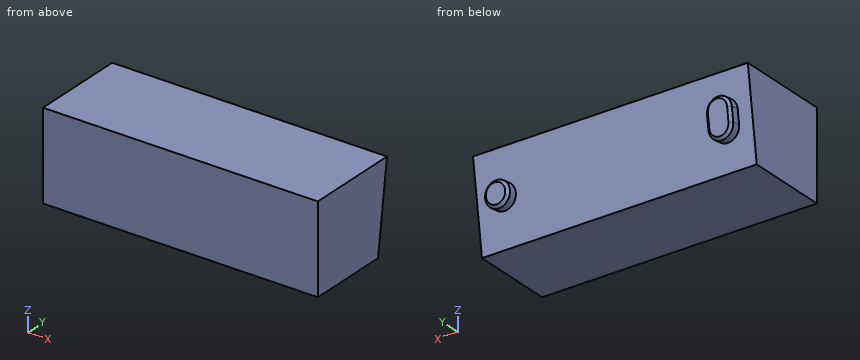
from build123d import *

# Parameters (mm, degrees)
EXTRUDE_1_DEPTH     = 16
CUT_EXTRUDE_1_DEPTH = 50
EXTRUDE_2_DEPTH     = 28.5
SKETCH_4_R          = 4.5
CUT_EXTRUDE_2_DEPTH = 28.5
EXTRUDE_3_DEPTH     = 50
EXTRUDE_START       = 4
SKETCH_6_R          = 4.5
EXTRUDE_4_DEPTH     = 4
CUT_EXTRUDE_3_DEPTH = 60
CHAMFER_1_SIZE      = 1


with BuildPart() as part:
    # 草图1 → 凸台-拉伸1 (new, symmetric)
    with BuildSketch(Plane.XY):
        with BuildLine():
            Line((-17, 0), (-17, -66.86388681))
            Line((-17, -66.86388681), (-20.5, -66.86388681))
            Line((-20.5, -66.86388681), (-20.5, 0))
            ThreePointArc((-20.5, 0), (0, 20.5), (20.5, 0))
            Line((20.5, 0), (20.5, -66.86388681))
            Line((20.5, -66.86388681), (17, -66.86388681))
            Line((17, -66.86388681), (17, 0))
            ThreePointArc((17, 0), (0, 17), (-17, 0))
        make_face()
    extrude(amount=EXTRUDE_1_DEPTH, both=True)

    # 草图2 → 切除-拉伸1 (cut, symmetric)
    with BuildSketch(Plane(origin=(0, 0, 0), x_dir=(0, 0, -1), z_dir=(1, 0, 0))):
        Polygon((16, -42.748653355), (-16, -38.251346645), (-16, -66.86388681), (16, -66.86388681), align=None)
    extrude(amount=CUT_EXTRUDE_1_DEPTH, both=True, mode=Mode.SUBTRACT)

    # 草图3 → 凸台-拉伸2 (add)
    with BuildSketch(Plane.ZY.offset(20.5)):
        Polygon((-16, -42.748653355), (16, -38.251346645), (16, -34.716950141), (-16, -39.214256851), align=None)
    extrude_2 = extrude(amount=EXTRUDE_2_DEPTH)

    # 镜向1: 凸台-拉伸2 across plane
    add(extrude_2.mirror(Plane(origin=(0, 0, 0), x_dir=(0, 0, 1), z_dir=(1, 0, 0))))

    # 草图4 → 切除-拉伸2 (cut)
    with BuildSketch(Plane(origin=(0, -36.249611102, 5.094550602), x_dir=(1, 0, 0), z_dir=(0, 0.9902680687415715, -0.13917310096005808))):
        with Locations(Location((40.5, 5.144617667, 0), (0, 0, 270))):
            Circle(SKETCH_4_R)
        with BuildLine():
            Line((-36, 7.644617667), (-36, 2.644617667))
            ThreePointArc((-36, 2.644617667), (-40.5, -1.855382333), (-45, 2.644617667))
            Line((-45, 2.644617667), (-45, 7.644617667))
            ThreePointArc((-45, 7.644617667), (-40.5, 12.144617667), (-36, 7.644617667))
        make_face()
    extrude(amount=-CUT_EXTRUDE_2_DEPTH, mode=Mode.SUBTRACT)

    # 草图8 → 切除-拉伸3 (cut, symmetric)
    with BuildSketch(Plane(origin=(0, 0, 0), x_dir=(0, 0, -1), z_dir=(1, 0, 0))):
        Polygon((16, -42.748653355), (-16, -38.251346645), (-16, 32.293524638), (16, 32.293524638), align=None)
    extrude(amount=CUT_EXTRUDE_3_DEPTH, both=True, mode=Mode.SUBTRACT)


with BuildPart() as body_2:
    # 草图5 → 凸台-拉伸3 (new, symmetric)
    with BuildSketch(Plane(origin=(0, 0, 0), x_dir=(0, 0, -1), z_dir=(1, 0, 0))):
        Polygon((16, -42.748653355), (-16, -38.251346645), (-16, -72.998653355), (16, -72.998653355), align=None)
    extrude(amount=EXTRUDE_3_DEPTH, both=True)

    # 草图6 → 凸台-拉伸4 (add)
    with BuildSketch(Plane(origin=(0, -39.715549343, 5.581656455), x_dir=(1, 0, 0), z_dir=(0, 0.9902680687415714, -0.139173100960058)).offset(EXTRUDE_START)):
        with Locations(Location((40.5, 5.144617667, 0), (0, 0, 90))):
            Circle(SKETCH_6_R)
        with BuildLine():
            Line((-36, 2.644617667), (-36, 7.644617667))
            ThreePointArc((-36, 7.644617667), (-40.5, 12.144617667), (-45, 7.644617667))
            Line((-45, 7.644617667), (-45, 2.644617667))
            ThreePointArc((-45, 2.644617667), (-40.5, -1.855382333), (-36, 2.644617667))
        make_face()
    extrude(amount=-EXTRUDE_4_DEPTH)

    # 倒角1
    chamfer_1_edges = [body_2.edges().sort_by_distance(p)[0] for p in [
        (-40.5, -35.496257755, 6.862289931),
        (-36, -36.470469462, -0.06958655),
        (-40.5, -37.444681169, -7.001463032),
        (-45, -36.470469462, -0.06958655),
        (40.5, -35.844190507, 4.386619759),
    ]]
    chamfer(chamfer_1_edges, length=CHAMFER_1_SIZE)


solid = body_2.part
Input: part model. Units: mm. Frame: model coordinates. Give positions to 0.01 mm unless a question says otherwise; leave off trailing zeros. Order: outer loops, then holes, each group sorted by start corner. A loop starts at its lowest first (then second) coordinate and runs counter-clockwise, first axis right, second up. Notation, with made-up numbers: (65, 63) -> (72, 63) arc R14 ccw to (72, 90) -> close; hole circle Ø1 at (80.5, -27.75). An arc over 180 degrees is marked (long way). Use one line per item in the form item = value.
1) Line query: probe 1 along Y at (x, z) = (-31.5, -4); probe 2 along Y at (x, z) = (18, -6.5). Output: solid intervals per line, ascending.
Response values:
probe_1 = -73 to -41.06
probe_2 = -73 to -41.41
2) First-contact query: pin 1 Ø12 at (x, z) = (22.5, -1.5) entering from +Y; pin 2 Ø10 at (x, z) = (-21.5, 0.5) entering from +Y; pin 3 Ø10 at (x, z) = (32.5, 6) entering from +Y. Flat tips, straight axial feed; report the tip coordinate or a pass-through.
Response values:
pin_1 = -39.87
pin_2 = -39.73
pin_3 = -38.95
3) Section A-A, the plane x = 11. Return loops of the section in (y, z), and give its area (3 significant figures).
Response values:
outline = (-73, -16) -> (-42.75, -16) -> (-38.25, 16) -> (-73, 16) -> close
area = 1,040 mm^2
4) Section B-B, the plane z = -8. Return loops of the section in (x, y), and give its area (3 significant figures).
Response values:
outline = (-50, -73) -> (50, -73) -> (50, -41.62) -> (-50, -41.62) -> close
area = 3,140 mm^2
